The listing builds one solid part. Answer for the finished solid, in the listing's coordinates (mm). Face numbers are marked on the shaded views. A direction names the side the tool comes from. Coordinates: 2 decimals unless noted, no trailing zeros. Order: outer loops, then holes, each group sorted by start corner. A loop starts at its lowest first (then second) coordinate and runs counter-clockwise, first axis right, second up.
from build123d import *

# Parameters (mm, degrees)
F1_DEPTH = 3.81
F2_R     = 3.81
F3_DEPTH = 10.414
F5_D     = 2.54
F5_DEPTH = 12.7
F5_TIP   = 0.7630929862


with BuildPart() as f1:
    # F0 (on Top) → F1 (new body)
    with BuildSketch(Plane.XY):
        with BuildLine():
            Line((0, 93.98), (0, 5.08))
            ThreePointArc((0, 5.08), (5.08, 0), (10.16, 5.08))
            Line((10.16, 5.08), (10.16, 93.98))
            ThreePointArc((10.16, 93.98), (5.08, 99.06), (0, 93.98))
        make_face()
    extrude(amount=F1_DEPTH)

    # F2 (on face) → F3 (join)
    with BuildSketch(Plane.XY.offset(3.81)):
        with Locations((5.08, 5.08)):
            Circle(F2_R)
    extrude(amount=F3_DEPTH)

    # F5
    with Locations(Plane.XY.offset(14.224)):
        with Locations((5.08, 5.08)):
            Hole(F5_D / 2, depth=F5_DEPTH)
            with Locations((0, 0, -(F5_DEPTH + F5_TIP / 2))):  # 118° drill point
                Cone(0, F5_D / 2, F5_TIP, mode=Mode.SUBTRACT)


solid = f1.part
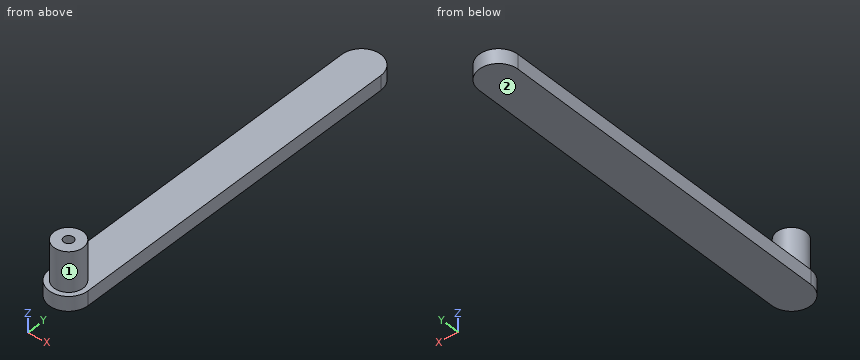
(1) Given pin 1 Ø3 at (x, y) = (4, 32.5) entering from +Z, flat-ended and moving along its own axis, determine where the tip first touches the part or whether it passes through.
(2) A tool of negligible diameter and unlimited length cuts with its end or side. For the marked faces 1 and 2, from which of +Z, -Z, +X, -X, +Y, -Y can it reach the whole face along a straight path? Write none if from no direction.
(3) Find section C-C on y = 49. Determine the outline of the cut face in (x, z).
(4) Find section B-B on x = 8. Determine the outline of the cut face in (y, z), then the cut area to 3 significant figures.
(5) Find the intervals of material crossed by probe 1 along Y at (x, z) = (5.08, 11.25); probe 2 along Z at (x, y) = (9, 47); probe 3 along Y at (x, z) = (6, 8.75), in increasing order.
(6) Find section A-A on z = 11. Determine the outline of the cut face in (x, y).
Resolved:
1. pin 1: stops at z = 3.81
2. face 1: +Z
2. face 2: -Z, +X, -X, +Y, -Y
3. outline: (0, 0) - (10.16, 0) - (10.16, 3.81) - (0, 3.81) - close
4. outline: (0.92, 0) - (98.14, 0) - (98.14, 3.81) - (7.53, 3.81) - (7.53, 14.22) - (2.63, 14.22) - (2.63, 3.81) - (0.92, 3.81) - close
4. area: 421 mm2
5. probe 1: y = 1.27 to 3.81, 6.35 to 8.89
5. probe 2: z = 0 to 3.81
5. probe 3: y = 1.38 to 4.2, 5.96 to 8.78
6. outline: circle Ø7.62 at (5.08, 5.08); hole circle Ø2.54 at (5.08, 5.08)
